```python
from build123d import *

# Parameters (mm, degrees)
SKETCH_3_W           = 36
SKETCH_3_H           = 50
EXTRUDE_1_DEPTH      = 24
SKETCH_4_W           = 24.8
SKETCH_4_H           = 31.8
CUT_EXTRUDE_1_DEPTH  = 19.7
SKETCH_5_W           = 14
SKETCH_5_H           = 2.2
CUT_EXTRUDE_3_DEPTH  = 19.7
SKETCH_6_W           = 18.5
SKETCH_6_H           = 3.8
CUT_EXTRUDE_4_DEPTH  = 14.7
SKETCH_7_W           = 24.8
SKETCH_7_H           = 24.280407208
CUT_EXTRUDE_5_DEPTH  = 2
SKETCH_8_R           = 2
CUT_EXTRUDE_6_DEPTH  = 6.4
SKETCH_9_R           = 1
CUT_EXTRUDE_7_DEPTH  = 6.4
SKETCH_10_R          = 2
CUT_EXTRUDE_8_DEPTH  = 7.4
SKETCH_11_R          = 1
CUT_EXTRUDE_9_DEPTH  = 7.4
SKETCH_14_W          = 47.693248889
SKETCH_14_H          = 41.94352182
CUT_EXTRUDE_12_DEPTH = 4
SKETCH_16_W          = 69.166934332
SKETCH_16_H          = 39.422219991
CUT_EXTRUDE_13_DEPTH = 5
CUT_EXTRUDE_17_DEPTH = 19.7
SKETCH_19_W          = 18.6
SKETCH_19_H          = 1.8
CUT_EXTRUDE_18_DEPTH = 12.7
SKETCH_20_W          = 66.697030433
SKETCH_20_H          = 63.084499434
CUT_EXTRUDE_19_DEPTH = 3.15
SKETCH_21_W          = 24.8
SKETCH_21_H          = 17.7
CUT_EXTRUDE_20_DEPTH = 10
SKETCH_22_W          = 12
SKETCH_22_H          = 15
SKETCH_22_R          = 1.6
EXTRUDE_2_DEPTH      = 2.9
SKETCH_23_W          = 25.2
SKETCH_23_H          = 39.225239964
CUT_EXTRUDE_22_DEPTH = 19.7
SKETCH_24_W          = 25.2
SKETCH_24_H          = 2.9
CUT_EXTRUDE_23_DEPTH = 4.3
FILLET_1_R           = 3


with BuildPart() as part:
    # 草图3 → 凸台-拉伸1 (new body)
    with BuildSketch(Plane(origin=(0, 0, 0), x_dir=(1, 0, 0), z_dir=(0, 1, 0))):
        Rectangle(SKETCH_3_W, SKETCH_3_H)
    extrude(amount=EXTRUDE_1_DEPTH)

    # 草图4 → 切除-拉伸1 (cut)
    with BuildSketch(Plane(origin=(0, 24, 0), x_dir=(1, 0, 0), z_dir=(0, 1, 0))):
        Rectangle(SKETCH_4_W, SKETCH_4_H)
    extrude(amount=-CUT_EXTRUDE_1_DEPTH, mode=Mode.SUBTRACT)

    # 草图5 → 切除-拉伸3 (cut)
    with BuildSketch(Plane(origin=(0, 24, 0), x_dir=(1, 0, 0), z_dir=(0, 1, 0))):
        with Locations((0, 15.9)):
            Rectangle(SKETCH_5_W, SKETCH_5_H)
    extrude(amount=-CUT_EXTRUDE_3_DEPTH, mode=Mode.SUBTRACT)

    # 草图6 → 切除-拉伸4 (cut)
    with BuildSketch(Plane(origin=(0, 24, 0), x_dir=(1, 0, 0), z_dir=(0, 1, 0))):
        with Locations((0, -15.9)):
            Rectangle(SKETCH_6_W, SKETCH_6_H)
    extrude(amount=-CUT_EXTRUDE_4_DEPTH, mode=Mode.SUBTRACT)

    # 草图7 → 切除-拉伸5 (cut)
    with BuildSketch(Plane(origin=(0, 24, 0), x_dir=(1, 0, 0), z_dir=(0, 1, 0))):
        with Locations((0, -25)):
            Rectangle(SKETCH_7_W, SKETCH_7_H)
    extrude(amount=-CUT_EXTRUDE_5_DEPTH, mode=Mode.SUBTRACT)

    # 草图8 → 切除-拉伸6 (cut)
    with BuildSketch(Plane.XY.offset(25)):
        with Locations((10.65, 7.2)):
            Circle(SKETCH_8_R)
        with Locations((-10.65, 7.2)):
            Circle(SKETCH_8_R)
    extrude(amount=-CUT_EXTRUDE_6_DEPTH, mode=Mode.SUBTRACT)

    # 草图9 → 切除-拉伸7 (cut)
    with BuildSketch(Plane.XY.offset(18.6)):
        with Locations((10.65, 7.2)):
            Circle(SKETCH_9_R)
        with Locations((-10.65, 7.2)):
            Circle(SKETCH_9_R)
    extrude(amount=-CUT_EXTRUDE_7_DEPTH, mode=Mode.SUBTRACT)

    # 草图10 → 切除-拉伸8 (cut)
    with BuildSketch(Plane(origin=(0, 0, -25), x_dir=(-1, 0, 0), z_dir=(0, 0, -1))):
        with Locations((-10.565, 11)):
            Circle(SKETCH_10_R)
        with Locations((10.56, 11)):
            Circle(SKETCH_10_R)
    extrude(amount=-CUT_EXTRUDE_8_DEPTH, mode=Mode.SUBTRACT)

    # 草图11 → 切除-拉伸9 (cut)
    with BuildSketch(Plane(origin=(0, 0, -17.6), x_dir=(-1, 0, 0), z_dir=(0, 0, -1))):
        with Locations((10.56, 11)):
            Circle(SKETCH_11_R)
        with Locations((-10.565, 11)):
            Circle(SKETCH_11_R)
    extrude(amount=-CUT_EXTRUDE_9_DEPTH, mode=Mode.SUBTRACT)

    # 草图14 → 切除-拉伸12 (cut)
    with BuildSketch(Plane.XY.offset(25)):
        with Locations((-2.653720185, 12.393348568)):
            Rectangle(SKETCH_14_W, SKETCH_14_H)
    extrude(amount=-CUT_EXTRUDE_12_DEPTH, mode=Mode.SUBTRACT)

    # 草图16 → 切除-拉伸13 (cut)
    with BuildSketch(Plane(origin=(0, 0, -25), x_dir=(-1, 0, 0), z_dir=(0, 0, -1))):
        with Locations((0.858826259, 12.588310345)):
            Rectangle(SKETCH_16_W, SKETCH_16_H)
    extrude(amount=-CUT_EXTRUDE_13_DEPTH, mode=Mode.SUBTRACT)

    # 草图18 → 切除-拉伸17 (cut)
    with BuildSketch(Plane(origin=(0, 24, 0), x_dir=(1, 0, 0), z_dir=(0, 1, 0))):
        Polygon((-12.6, -16.1), (12.6, -16.1), (12.6, 16.1), (7.2, 16.1), (7.2, 17.2), (-7.2, 17.2), (-7.2, 16.1), (-12.6, 16.1), align=None)
    extrude(amount=-CUT_EXTRUDE_17_DEPTH, mode=Mode.SUBTRACT)

    # 草图19 → 切除-拉伸18 (cut)
    with BuildSketch(Plane(origin=(0, 22, 0), x_dir=(1, 0, 0), z_dir=(0, 1, 0))):
        with Locations((0, -16.95)):
            Rectangle(SKETCH_19_W, SKETCH_19_H)
    extrude(amount=-CUT_EXTRUDE_18_DEPTH, mode=Mode.SUBTRACT)

    # 草图20 → 切除-拉伸19 (cut)
    with BuildSketch(Plane.XY.offset(21)):
        with Locations((4.746063078, 3.342697103)):
            Rectangle(SKETCH_20_W, SKETCH_20_H)
    extrude(amount=-CUT_EXTRUDE_19_DEPTH, mode=Mode.SUBTRACT)

    # 草图21 → 切除-拉伸20 (cut)
    with BuildSketch(Plane.XY.offset(17.85)):
        with Locations((0, 13.15)):
            Rectangle(SKETCH_21_W, SKETCH_21_H)
    extrude(amount=-CUT_EXTRUDE_20_DEPTH, mode=Mode.SUBTRACT)

    # 草图22 → 凸台-拉伸2 (add)
    with BuildSketch(Plane.XY.offset(17.85)):
        with Locations((18.4, 7.5)):
            Rectangle(SKETCH_22_W, SKETCH_22_H)
        with Locations((21.9, 7.5)):
            Circle(SKETCH_22_R, mode=Mode.SUBTRACT)
    extrude_2 = extrude(amount=EXTRUDE_2_DEPTH)

    # 镜向1: 凸台-拉伸2 across plane
    add(extrude_2.mirror(Plane(origin=(0, 0, 0), x_dir=(0, 0, 1), z_dir=(1, 0, 0))))

    # 草图23 → 切除-拉伸22 (cut)
    with BuildSketch(Plane(origin=(0, 24, 0), x_dir=(1, 0, 0), z_dir=(0, 1, 0))):
        with Locations((0, -3.512619982)):
            Rectangle(SKETCH_23_W, SKETCH_23_H)
    extrude(amount=-CUT_EXTRUDE_22_DEPTH, mode=Mode.SUBTRACT)

    # 草图24 → 切除-拉伸23 (cut)
    with BuildSketch(Plane(origin=(0, 4.3, 0), x_dir=(1, 0, 0), z_dir=(0, 1, 0))):
        with Locations((0, -19.3)):
            Rectangle(SKETCH_24_W, SKETCH_24_H)
    extrude(amount=-CUT_EXTRUDE_23_DEPTH, mode=Mode.SUBTRACT)

    # 圆角1
    fillet_1_edges = [part.edges().sort_by_distance(p)[0] for p in [
        (-18, 12, -20),
        (18, 12, -20),
    ]]
    fillet(fillet_1_edges, radius=FILLET_1_R)


solid = part.part
```
Model file for the job. Use its own axes, mm. A direction names the side the tool comes from. Round coordinates to 2 decimals unless told otherwise and drop trailing zeros. Write each loop counter-clockwise with the first axis right and the second up, starting at its lowest first coordinate (ties: lowest second). Pieces come first, ordered by that corner, then holes. Notation, with made-up numbers: M 80,9 L 84,9 A15 ccw 84,25 Z; hole C 55.25,-16.75 d11. An arc over 180 degrees is marked long. Put each result on its own line as item: value.
Item 1: Cut at A-A (y = 11). State how many separate pieces and enclosed holes the cut face has, and give its area (3 significant figures).
Responses:
separate pieces: 3
enclosed holes: 0
area: 531 mm²
Item 2: Cut at B-B (x = 21.9). List the corners of the cut face in (y, z), and give its area (3 significant figures).
Responses:
outline: M 0,17.85 L 5.9,17.85 L 5.9,20.75 L 0,20.75 Z; M 9.1,17.85 L 15,17.85 L 15,20.75 L 9.1,20.75 Z
area: 34.2 mm²
Item 3: Flat gauge pins, fed straight in: P1, Ø12.5, axis at x = -2.5, z = -0.5, coming from the +Y side; P2, Ø1.2, axis at x = 11.5, y = 11, coming from the -Z side; P3, Ø3.5, axis at x = 2, y = 1, coming from the +Z side; P4, Ø1.2, axis at x = 10.565, y = 11, coming from the -Z side. Where does each tip first touch, or does it go through?
Responses:
P1: y = 4.3
P2: z = -17.6
P3: z = 17.85
P4: through
Item 4: Probe L1, parallel to X at y = 4.75, z = -1.5; L2, parallel to Y at x = -21.9, z = 20; L3, parallel to Z at x = -4, y = 21.5. List the from-to ranges inside material, lowest first. Write a range as from..to.
Responses:
L1: -18..-12.6, 12.6..18
L2: 0..5.9, 9.1..15
L3: -20..-17.2
Item 5: Mould opens along Y. For faces 6 (the flat face through (-18, 15, 19)), 7 (the flat face through (0, 14, -17.2)), 8 (the cylindrical face through (-11.484, 10.617, -16.86)) say: +Y half, -Y half, draft (parallel to the pull), parting line (faces both ways), or undercut.
Responses:
face 6: +Y half
face 7: draft
face 8: undercut
Item 6: Cut at D-D (z = 1). List the corners of the cut face in (x, y), and give its area (3 significant figures).
Responses:
outline: M -18,0 L 18,0 L 18,24 L 12.6,24 L 12.6,4.3 L -12.6,4.3 L -12.6,24 L -18,24 Z
area: 368 mm²
Item 7: Tool access for faces 1 (the flat face through (-20, 8, 17.85)), 2 (the flat face through (-15, 20, 17.85)), 3 (the flat face through (-10, 14, -16.1)), 4 (the flat face through (18, 12, 1)), 5 (the flat face through (9.7, 10.1, -17.6)): list every direction of +Z, -Z, +X, -X, +Y, -Y with a clear straight run to the whole face (end or side of a thin tool).
Responses:
face 1: -Z, -X, +Y, -Y
face 2: +Z, +X, -X, +Y
face 3: +Z, +Y
face 4: -Z, +X, +Y, -Y
face 5: -Z
Item 8: Cut at C-C (y = 15.75). List the corners of the cut face in (x, z), and give its area (3 significant figures).
Responses:
outline: M -18,-17 A3 ccw -15,-20 L 15,-20 A3 ccw 18,-17 L 18,17.85 L 12.6,17.85 L 12.6,-16.1 L 7.2,-16.1 L 7.2,-17.2 L -7.2,-17.2 L -7.2,-16.1 L -12.6,-16.1 L -12.6,17.85 L -18,17.85 Z
area: 487 mm²
